The listing builds one solid part. Answer for the finished solid, in the listing's coordinates (mm). Face numbers are marked on the shaded views. A direction names the side the tool comes from. Give positions to 0.01 mm unless a question says otherwise; leave off trailing zeros. Order: outer loops, then holes, each group sorted by start corner. A loop starts at its lowest first (then second) coordinate and runs counter-clockwise, first axis right, second up. Notation, with made-up numbers: (38, -1) - (49, -1) arc R15 cw to (49, 10) - close; hole circle Ø6 at (34, -10). An arc over 180 degrees is marked (long way). Use CSV: the item, a comma, the result in double quotes.
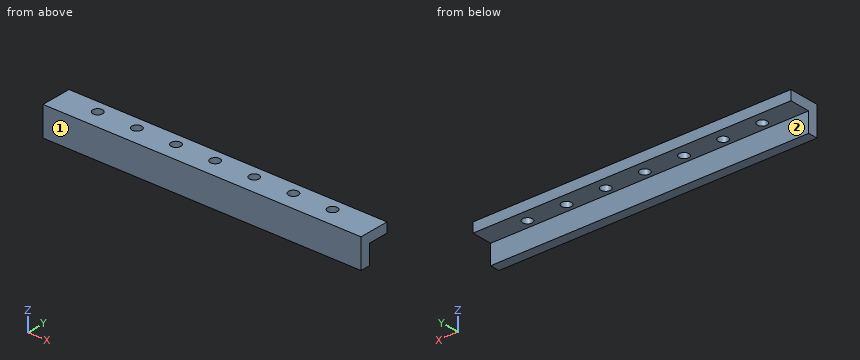
```python
from build123d import *

# Parameters (mm, degrees)
BOSS_EXTRUDE1_DEPTH = 206.375
SKETCH2_R           = 3.175
CUT_EXTRUDE1_DEPTH  = 209.19716249
LPATTERN1_COUNT     = 7
LPATTERN1_PITCH     = 25.4


with BuildPart() as part:
    # Sketch1 → Boss-Extrude1 (new body)
    with BuildSketch(Plane(origin=(0, 0, 0), x_dir=(0, 0, -1), z_dir=(1, 0, 0))):
        Polygon((0, 0), (0, 19.812), (6.35, 19.812), (6.35, 6.35), (19.05, 6.35), (19.05, 0), align=None)
    extrude(amount=BOSS_EXTRUDE1_DEPTH)

    # Sketch2 → Cut-Extrude1 (cut, through all)
    with BuildSketch(Plane.XY):
        with Locations((25.4, 11.8745)):
            Circle(SKETCH2_R)
    cut_extrude1 = extrude(amount=-CUT_EXTRUDE1_DEPTH, mode=Mode.SUBTRACT)

    # LPattern1: Cut-Extrude1 ×7
    with Locations(*[(i * LPATTERN1_PITCH, 0, 0) for i in range(1, LPATTERN1_COUNT)]):
        add(cut_extrude1, mode=Mode.SUBTRACT)


solid = part.part
```
Item 1: The part is cut by section A-A (x = 76.2). Give the vertices of the cut face in (y, z), and give its area (3 significant figures).
Taken from the geometry:
outline,"(0, -19.05) - (6.35, -19.05) - (6.35, -6.35) - (8.7, -6.35) - (8.7, 0) - (0, 0) - close; (15.05, -6.35) - (19.81, -6.35) - (19.81, 0) - (15.05, 0) - close"
area,"166 mm^2"
Item 2: Which of the six approach directions +Z, -Z, +X, -X, +Y, -Y give full straight-line access (tool end or side, diameter ignored) to the marked faces 1 and 2?
Taken from the geometry:
face 1,"+Z, -Z, +X, -X, -Y"
face 2,"-Z, +X, -X, +Y"
Item 3: The part is cut by section B-B (x = 142.5). Give the vertices of the cut face in (y, z).
Taken from the geometry:
outline,"(0, -19.05) - (6.35, -19.05) - (6.35, -6.35) - (19.81, -6.35) - (19.81, 0) - (0, 0) - close"
Item 4: Find the intervals of material crossed by line 1 along Y through (x, z) = (152.4, -1.75); line 2 along Y through (x, z) = (104, -14.5); line 3 along Z through (x, y) = (150, 7.5), in increasing order.
Taken from the geometry:
line 1,"0 to 8.7, 15.05 to 19.81"
line 2,"0 to 6.35"
line 3,"-6.35 to 0"
Item 5: Each of these flat-tipped pins is pushed along its axis until it touches: pin 1 (10 mm diameter, centred on x = 76.2, y = 11.87, fed in from -Z); pin 2 (3 mm diameter, centred on x = 128, z = -9, fed in from +Y). Where does it stop, or does it pass through?
Taken from the geometry:
pin 1,"z = -6.35"
pin 2,"y = 6.35"
Item 6: The part is cut by section C-C (z = -16.75). Give the vertices of the cut face in (x, y) (3 decimals), and give its area (3 significant figures).
Taken from the geometry:
outline,"(0, 0) - (206.375, 0) - (206.375, 6.35) - (0, 6.35) - close"
area,"1,310 mm^2"
